Read the model definition and answer for the solid it produces. Units are mm, in the model's axes. Coordinates: 2 decimals unless noted, no trailing zeros. Loops run counter-clockwise (first coordinate to the right, second up) from the corner with the lowest first, then second, coordinate; pieces in that order, holes last. Notation, with made-up numbers: (6, 29.5) - (47, 29.5) arc R34 ccw to (47, 67.5) - close; hole circle Ø9 at (2, 44.25). An arc over 180 degrees is marked (long way). Use one line per item in the form item = value.
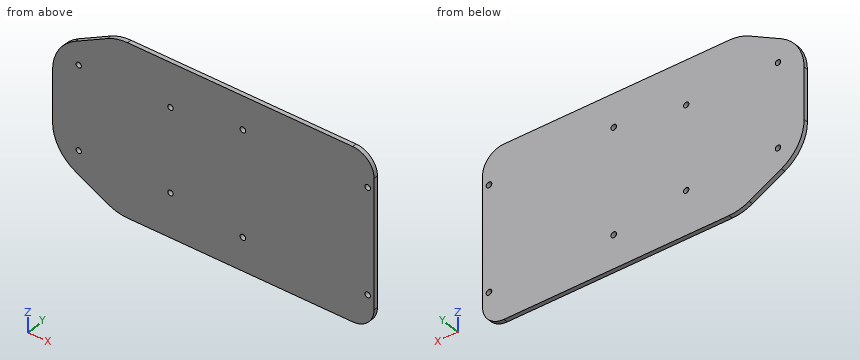
from build123d import *

# Parameters (mm, degrees)
SKETCH_1_W          = 150
SKETCH_1_H          = 80
SKETCH_1_R          = 1.25
EXTRUDE_1_DEPTH     = 2
SKETCH_2_R          = 1.3
CUT_EXTRUDE_1_DEPTH = 2
CUT_EXTRUDE_2_DEPTH = 2
FILLET_1_R          = 20
FILLET_2_R          = 10


with BuildPart() as part:
    # 草图1 → 凸台-拉伸1 (new body)
    with BuildSketch(Plane(origin=(0, 0, 0), x_dir=(1, 0, 0), z_dir=(0, 1, 0))):
        Rectangle(SKETCH_1_W, SKETCH_1_H)
        with Locations(Location((-62.8, 19.5, 0), (0, 0, 270))):
            Circle(SKETCH_1_R, mode=Mode.SUBTRACT)
        with Locations(Location((-20, 19.5, 0), (0, 0, 90))):
            Circle(SKETCH_1_R, mode=Mode.SUBTRACT)
        with Locations(Location((-20, -19.5, 0), (0, 0, 270))):
            Circle(SKETCH_1_R, mode=Mode.SUBTRACT)
        with Locations(Location((-62.8, -19.5, 0), (0, 0, 90))):
            Circle(SKETCH_1_R, mode=Mode.SUBTRACT)
    extrude(amount=EXTRUDE_1_DEPTH)

    # 草图2 → 切除-拉伸1 (cut)
    with BuildSketch(Plane(origin=(0, 2, 0), x_dir=(1, 0, 0), z_dir=(0, 1, 0))):
        with Locations(Location((13.8, 24.5, 0), (0, 0, 270))):
            Circle(SKETCH_2_R)
        with Locations(Location((72, 24.5, 0), (0, 0, 90))):
            Circle(SKETCH_2_R)
        with Locations(Location((13.8, -24.5, 0), (0, 0, 90))):
            Circle(SKETCH_2_R)
        with Locations(Location((72, -24.5, 0), (0, 0, 270))):
            Circle(SKETCH_2_R)
    extrude(amount=-CUT_EXTRUDE_1_DEPTH, mode=Mode.SUBTRACT)

    # 草图3 → 切除-拉伸2 (cut)
    with BuildSketch(Plane(origin=(0, 2, 0), x_dir=(1, 0, 0), z_dir=(0, 1, 0))):
        Polygon((-75, 40), (-45, 40), (-75, 24), align=None)
        Polygon((-45, -40), (-75, -24), (-75, -40), align=None)
    extrude(amount=-CUT_EXTRUDE_2_DEPTH, mode=Mode.SUBTRACT)

    # 圆角1
    fillet_1_edges = [part.edges().sort_by_distance(p)[0] for p in [
        (-75, 1, -24),
        (-45, 1, -40),
        (-45, 1, 40),
        (-75, 1, 24),
    ]]
    fillet(fillet_1_edges, radius=FILLET_1_R)

    # 圆角2
    fillet_2_edges = [part.edges().sort_by_distance(p)[0] for p in [
        (75, 1, 40),
        (75, 1, -40),
    ]]
    fillet(fillet_2_edges, radius=FILLET_2_R)


solid = part.part
Item 1: Find the intervals of material crossed by L1, parallel to X at y = 0.45, z = 19.5; L2, parallel to Z at x = 72, y = 0.9; L3, parallel to X at y = 1.15, z = 24.5, in increasing order.
Results below:
L1 = -73.54 to -64.05, -61.55 to -21.25, -18.75 to 75
L2 = -37.14 to -25.8, -23.2 to 23.2, 25.8 to 37.14
L3 = -70.61 to 12.5, 15.1 to 70.7, 73.3 to 75
Item 2: The part is cut by section A-A on y = 1. Count the separate pieces of the cut face and the enclosed holes in it, plus the area to 3 significant figures.
Results below:
separate_pieces = 1
enclosed_holes = 8
area = 11,400 mm²
Item 3: This flat-tipped pin is pushed along its axis until it touches: P1, Ø2, axis at x = -62.8, z = 19.5, coming from the +Y side. Where does it stop, or does it pass through?
Results below:
P1 = through
Item 4: The part is cut by section B-B on x = -52. Give the vertices of the cut face in (y, z), plus the area to 3 significant figures.
Results below:
outline = (0, -36.27) - (2, -36.27) - (2, 36.27) - (0, 36.27) - close
area = 145 mm²
